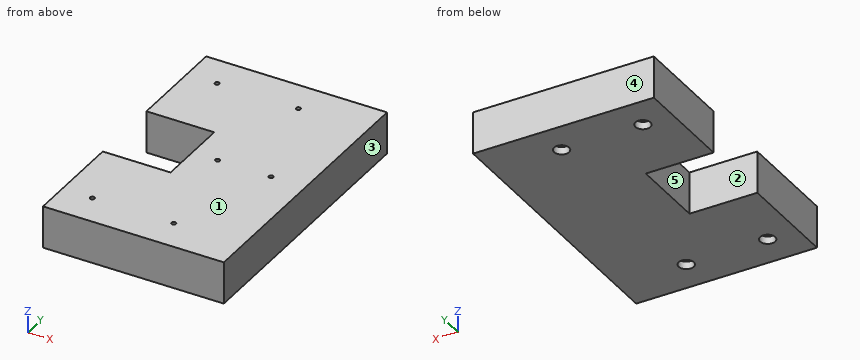
from build123d import *

# Parameters (mm, degrees)
SKETCH_W         = 120
SKETCH_H         = 28
PAD_DEPTH        = 93.3
SKETCH001_R      = 1.5
POCKET_DEPTH     = 10
HOLE_D           = 3
HOLE_CBORE_D     = 10
HOLE_CBORE_DEPTH = 5
SKETCH003_W      = 45
SKETCH003_H      = 50
POCKET001_DEPTH  = 28.001


with BuildPart() as part:
    # Sketch → Pad (new body, symmetric)
    with BuildSketch(Plane.XZ):
        Rectangle(SKETCH_W, SKETCH_H)
    extrude(amount=PAD_DEPTH, both=True)

    # Sketch001 (on Face1 of Pad) → Pocket (cut)
    with BuildSketch(Plane(origin=(0, 0, 14), x_dir=(-1, 0, 0), z_dir=(0, 0, 1))):
        with Locations((-37.25, 0)):
            Circle(SKETCH001_R)
        with Locations((-1.75, 0)):
            Circle(SKETCH001_R)
    extrude(amount=-POCKET_DEPTH, mode=Mode.SUBTRACT)

    # Hole (through all)
    with Locations(Plane(origin=(0, 0, -14), x_dir=(1, 0, 0), z_dir=(0, 0, -1))):
        with Locations((-40, 71.3), (14, 71.3), (14, -71.3), (-40, -71.3)):
            CounterBoreHole(HOLE_D / 2, HOLE_CBORE_D / 2, HOLE_CBORE_DEPTH)

    # Sketch003 (on Face1 of Hole) → Pocket001 (cut, through all)
    with BuildSketch(Plane(origin=(0, 0, 14), x_dir=(-1, 0, 0), z_dir=(0, 0, 1))):
        with Locations((37.5, 0)):
            Rectangle(SKETCH003_W, SKETCH003_H)
    extrude(amount=-POCKET001_DEPTH, mode=Mode.SUBTRACT)


solid = part.part
The model under review builds one solid part; all positions refer to its coordinate system, in mm. Face numbers are marked on the shaded views. A direction names the side the tool comes from. Round coordinates to 2 decimals unless told otherwise and drop trailing zeros. Loops run counter-clockwise (first coordinate to the right, second up) from the corner with the lowest first, then second, coordinate; pieces in that order, holes last. Notation, with made-up numbers: (38, 81.5) - (91, 81.5) arc R12 cw to (91, 94.5) - close; hole circle Ø4 at (35, 27). An arc over 180 degrees is marked (long way). Use CSV: the item, a comma, the result in double quotes.
(1) The part is to be moulded in two halves that separate along Y. For the marked faces 3, 4 and 5, say which applies: pulls with the +Y half, pulls with the -Y half, needs draft (parallel to the pull), parting line crosses it, or undercut.
Working result:
face 3,"needs draft"
face 4,"pulls with the +Y half"
face 5,"undercut"
(2) Take a section at C-C, the plane z = 9.25. Give the boundary of the cut face in (x, y).
Working result:
outline,"(-60, -93.3) - (60, -93.3) - (60, 93.3) - (-60, 93.3) - (-60, 25) - (-15, 25) - (-15, -25) - (-60, -25) - close; hole circle Ø3 at (-40, -71.3); hole circle Ø3 at (-40, 71.3); hole circle Ø3 at (1.75, 0); hole circle Ø3 at (14, -71.3); hole circle Ø3 at (14, 71.3); hole circle Ø3 at (37.25, 0)"
(3) Take a section at B-B, the plane z = -6. Give the boundary of the cut face in (x, y), plus the area to 3 significant figures.
Working result:
outline,"(-60, -93.3) - (60, -93.3) - (60, 93.3) - (-60, 93.3) - (-60, 25) - (-15, 25) - (-15, -25) - (-60, -25) - close; hole circle Ø3 at (-40, -71.3); hole circle Ø3 at (-40, 71.3); hole circle Ø3 at (14, -71.3); hole circle Ø3 at (14, 71.3)"
area,"20,100 mm^2"
(4) Clearance check with flat-ended pins moving along their axes: P1, Ø3, axis at x = 14.5, y = -71, coming from the -Z side; P2, Ø8, axis at y = -8, z = 10.5, coming from the -X side; P3, Ø2.5, axis at x = -40, y = -71.3, coming from the -Z side. State where each tip first meets the part, or that it passes through.
Working result:
P1,"stops at z = -9"
P2,"stops at x = -15"
P3,"passes through"
(5) For line 1 (Y direction, x = -40, z = -11); line 2 (X direction, y = -71.3, z = -3); line 3 (X direction, y = -71.3, z = -10.45), list the stretches that pass through material, from the lowest coordinate up.
Working result:
line 1,"y = -93.3 to -76.3, -66.3 to -25, 25 to 66.3, 76.3 to 93.3"
line 2,"x = -60 to -41.5, -38.5 to 12.5, 15.5 to 60"
line 3,"x = -60 to -45, -35 to 9, 19 to 60"
(6) Take a section at A-A, the plane x = -24. Give the boundary of the cut face in (y, z), plus the area to 3 significant figures.
Working result:
outline,"(-93.3, -14) - (-25, -14) - (-25, 14) - (-93.3, 14) - close; (25, -14) - (93.3, -14) - (93.3, 14) - (25, 14) - close"
area,"3,820 mm^2"
(7) Machinability: for the marked faces 1 and 2, which of the approach directions +Z, -Z, +X, -X, +Y, -Y give a long, thin tool a straight path to every point of the face, cutting with its end or side? Answer none if there is none.
Working result:
face 1,"+Z, +X, -X, +Y, -Y"
face 2,"+Z, -Z, -X"
